For this review, take the finished solid that the model builds, in its own axes (mm). A direction names the side the tool comes from. Coordinates: 2 decimals unless noted, no trailing zeros. Loops run counter-clockwise (first coordinate to the right, second up) from the corner with the lowest first, then second, coordinate; pieces in that order, holes last.
```python
from build123d import *

# Parameters (mm, degrees)
F0_W     = 215.1181101799
F0_H     = 210.1173847914
F1_DEPTH = 50.8
F2_R     = 53.1290592744
F3_DEPTH = 50.8
F3_TAPER = 10
F5_R     = 18.4483191982
F6_DEPTH = 25.4
F6_TAPER = 3


with BuildPart() as f1:
    # F0 (on Top) → F1 (new body)
    with BuildSketch(Plane.XY):
        Rectangle(F0_W, F0_H)
    extrude(amount=F1_DEPTH)

    # F2 (on face) → F3 (join)
    with BuildSketch(Plane.XY.offset(50.8)):
        Circle(F2_R)
    extrude(amount=F3_DEPTH, taper=F3_TAPER)

    # F5 (on face) → F6 (cut)
    with BuildSketch(Plane.XY.offset(101.6)):
        Circle(F5_R)
    extrude(amount=-F6_DEPTH, taper=F6_TAPER, mode=Mode.SUBTRACT)


solid = f1.part
```
Q1. Consider section D-D (x = -67). State the section outline as (y, z) points, then the cut area to 3 significant figures.
Q2. Consider section A-A (x = 0). State the section outline as (y, z) points, then the cut area to 3 significant figures.
Q3. Machinability: for faces 1 (the face through (107.559, -1, 25)), 2 (the face through (-25, 48, 50.8)), which of the approach directions +Z, -Z, +X, -X, +Y, -Y give a long, thin tool a straight path to every point of the face, cutting with its end or side? Answer none if there is none.
Q4. Wall thickness on probe 1 along Z at (x, y) = (79.5, -80); probe 2 along X at (y, z) = (-13.5, 64); probe 3 along Y at (x, z) = (-38, 75): over which ranges is each line inside the solid? List them lowest first.
Q5. Consider section C-C (z = 84). State the section outline as (x, y) points (3 decimals), then the cut area to 3 significant figures.
Q6. For pin 1 Ø10.5 at (x, y) = (-8, -6) entering from +Z; pin 2 Ø5 at (x, y) = (-24.5, -67.5) entering from +Z; pin 3 Ø4 at (x, z) = (-27.5, 82.5) entering from +Y; pin 4 Ø5 at (x, y) = (24, 66.5) entering from -Z, all flat-tipped, find the tip position at first contact; note any pin that passes through.
Q7. The part is to be moulded in two halves that separate along X. For faces 3 (the face through (8.2, -15.77, 88.72)), 4 (the face through (-2, -105.059, 25)), 5 (the face through (-107.559, -1, 25)), say which applies: +X half, -X half, draft (parallel to the pull), parting line (faces both ways), or undercut.
Q8. Consider section B-B (y = -73.5). State the section outline as (x, z) points.
Model answer:
1. outline: (-105.06, 0) - (105.06, 0) - (105.06, 50.8) - (-105.06, 50.8) - close
1. area: 10,700 mm2
2. outline: (-105.06, 0) - (105.06, 0) - (105.06, 50.8) - (53.13, 50.8) - (44.17, 101.6) - (18.45, 101.6) - (17.12, 76.2) - (-17.12, 76.2) - (-18.45, 101.6) - (-44.17, 101.6) - (-53.13, 50.8) - (-105.06, 50.8) - close
2. area: 14,700 mm2
3. face 1: +Z, -Z, +X, +Y, -Y
3. face 2: +Z
4. probe 1: z = 0 to 50.8
4. probe 2: x = -48.97 to 48.97
4. probe 3: y = -30.72 to 30.72
5. outline: circle Ø94.55 at (0, 0); hole circle Ø35.052 at (0, 0)
5. area: 6,060 mm2
6. pin 1: stops at z = 76.2
6. pin 2: stops at z = 50.8
6. pin 3: stops at y = 40.19
6. pin 4: stops at z = 0
7. face 3: undercut
7. face 4: draft
7. face 5: -X half
8. outline: (-107.56, 0) - (107.56, 0) - (107.56, 50.8) - (-107.56, 50.8) - close
